from build123d import *

# Parameters (mm, degrees)
CYLINDER001_R     = 1.8
CYLINDER001_DEPTH = 40
ARRAY002_X_COUNT  = 2
ARRAY002_X_PITCH  = 21
CYLINDER002_R     = 1
CYLINDER002_DEPTH = 100
ARRAY003_X_COUNT  = 2
ARRAY003_X_PITCH  = 43
ARRAY003_Y_COUNT  = 2
ARRAY003_Y_PITCH  = 72
CYLINDER003_R     = 1.8
CYLINDER003_DEPTH = 40
ARRAY004_Y_COUNT  = 2
ARRAY004_Y_PITCH  = 71
BOX005_W          = 4
BOX005_H          = 10
BOX005_DEPTH      = 40
CYLINDER004_R     = 2.2
CYLINDER004_DEPTH = 40
ARRAY005_Y_COUNT  = 2
ARRAY005_Y_PITCH  = 34
CYLINDER005_R     = 3
CYLINDER005_DEPTH = 40
CYLINDER_R        = 1.3
CYLINDER_DEPTH    = 40
ARRAY001_X_COUNT  = 2
ARRAY001_X_PITCH  = 19
BOX004_W          = 107
BOX004_H          = 80
BOX004_DEPTH      = 3
FILLET001_R       = 2


with BuildPart() as array002:
    # Cylinder001 → Cylinder001 (new body)
    with BuildSketch(Plane(origin=(75.5, 16.5, -15), x_dir=(1, 0, 0), z_dir=(0, 0, 1))):
        Circle(CYLINDER001_R)
    extrude(amount=CYLINDER001_DEPTH)

    # Array002 X: Array002 ×2


with BuildPart() as array002_1:
    add(array002.part)
    with Locations(*[(i * ARRAY002_X_PITCH, 0, 0) for i in range(1, ARRAY002_X_COUNT)]):
        add(array002.part)


with BuildPart() as array_battery_holder_holes:
    # Cylinder002 → Cylinder002 (new body)
    with BuildSketch(Plane(origin=(13, -4, -15), x_dir=(1, 0, 0), z_dir=(0, 0, 1))):
        Circle(CYLINDER002_R)
    extrude(amount=CYLINDER002_DEPTH)

    # Array003 X: Array battery holder holes ×2


with BuildPart() as array_battery_holder_holes_1:
    add(array_battery_holder_holes.part)
    with Locations(*[(i * ARRAY003_X_PITCH, 0, 0) for i in range(1, ARRAY003_X_COUNT)]):
        add(array_battery_holder_holes.part)

    # Array003 Y: Array battery holder holes ×2


with BuildPart() as array_battery_holder_holes_2:
    add(array_battery_holder_holes_1.part)
    with Locations(*[(0, i * ARRAY003_Y_PITCH, 0) for i in range(1, ARRAY003_Y_COUNT)]):
        add(array_battery_holder_holes_1.part)


with BuildPart() as array_corners:
    # Cylinder003 → Cylinder003 (new body)
    with BuildSketch(Plane(origin=(99, -4.5, -15), x_dir=(1, 0, 0), z_dir=(0, 0, 1))):
        Circle(CYLINDER003_R)
    extrude(amount=CYLINDER003_DEPTH)

    # Array004 Y: Array corners ×2


with BuildPart() as array_corners_1:
    add(array_corners.part)
    with Locations(*[(0, i * ARRAY004_Y_PITCH, 0) for i in range(1, ARRAY004_Y_COUNT)]):
        add(array_corners.part)


with BuildPart() as cube_switch_cut:
    # Box005 → Box005 (new body)
    with BuildSketch(Plane(origin=(78, 1.5, -10), x_dir=(0, -1, 0), z_dir=(0, 0, 1))):
        with Locations((2, 5)):
            Rectangle(BOX005_W, BOX005_H)
    extrude(amount=BOX005_DEPTH)


with BuildPart() as array_usb:
    # Cylinder004 → Cylinder004 (new body)
    with BuildSketch(Plane(origin=(91.5, 24.5, -15), x_dir=(1, 0, 0), z_dir=(0, 0, 1))):
        Circle(CYLINDER004_R)
    extrude(amount=CYLINDER004_DEPTH)

    # Array005 Y: Array usb ×2


with BuildPart() as array_usb_1:
    add(array_usb.part)
    with Locations(*[(0, i * ARRAY005_Y_PITCH, 0) for i in range(1, ARRAY005_Y_COUNT)]):
        add(array_usb.part)


with BuildPart() as cylinder_usb_center:
    # Cylinder005 → Cylinder005 (new body)
    with BuildSketch(Plane(origin=(86, 41.5, -15), x_dir=(1, 0, 0), z_dir=(0, 0, 1))):
        Circle(CYLINDER005_R)
    extrude(amount=CYLINDER005_DEPTH)


with BuildPart() as fusion001:
    # Cylinder → Cylinder (new body)
    with BuildSketch(Plane(origin=(73.5, -0.5, -15), x_dir=(0, -1, 0), z_dir=(0, 0, 1))):
        Circle(CYLINDER_R)
    extrude(amount=CYLINDER_DEPTH)

    # Array001 X: Fusion001 ×2


with BuildPart() as fusion001_1:
    add(fusion001.part)
    with Locations(*[(i * ARRAY001_X_PITCH, 0, 0) for i in range(1, ARRAY001_X_COUNT)]):
        add(fusion001.part)

    # Fusion001: union Array002, Array battery holder holes, Array corners, Cube switch cut, Array usb, Cylinder usb center
    add(array002_1.part)
    add(array_battery_holder_holes_2.part)
    add(array_corners_1.part)
    add(cube_switch_cut.part)
    add(array_usb_1.part)
    add(cylinder_usb_center.part)


with BuildPart() as top_lid_clone:
    # Box004 → Box004 (new body)
    with BuildSketch(Plane(origin=(-3, -8.5, -3), x_dir=(1, 0, 0), z_dir=(0, 0, 1))):
        with Locations((53.5, 40)):
            Rectangle(BOX004_W, BOX004_H)
    extrude(amount=BOX004_DEPTH)

    # Fillet001
    fillet001_edges = [top_lid_clone.edges().sort_by_distance(p)[0] for p in [
        (-3, -8.5, -1.5),
        (-3, 71.5, -1.5),
        (104, -8.5, -1.5),
        (104, 71.5, -1.5),
    ]]
    fillet(fillet001_edges, radius=FILLET001_R)

    # Cut001: cut Fusion001
    add(fusion001_1.part, mode=Mode.SUBTRACT)


solid = top_lid_clone.part
Source: CAD feature listing. Evaluate the final solid. Frame: model axes, mm. A direction names the side the tool comes from. Round coordinates to 2 decimals unless told otherwise and drop trailing zeros. Loops run counter-clockwise (first coordinate to the right, second up) from the corner with the lowest first, then second, coordinate; pieces in that order, holes last. Notation, with made-up numbers: (41, -14) - (75, -14) arc R17 cw to (75, 5) - close; hole circle Ø5 at (44.25, 39.5). An arc over 180 degrees is marked (long way). Write item = value, one per line. Start each with the question number.
Item 1: Reachability of faces 1 (the face through (83, -2.5, -2)), 2 (the face through (50, -8.5, -2)) from +Z, -Z, +X, -X, +Y, -Y: full face, straight path, thin tool, end or side. Return the list, or none.
Item 2: Section query B-B on y = 58.5. Output: boundary loops of the cut face in (x, z), plus the area to 3 significant figures.
Item 3: Material intervals for line 1 (Y direction, x = 99, z = -2.15); line 2 (Y direction, x = 13, z = -2.2); line 3 (Y direction, x = 91.5, z = -1.15), sorted ascending.
Item 4: Mould query, pull axis X, two halves, no side actions, for faces 3 (the face through (-3, 31, -2)), 4 (the face through (91.23, -0.22, -1.52)), 5 (the face through (50, 32, -3)). Classes: released by +X, released by -X, zero draft, split by the parting line, or undercut.
Item 5: Section query C-C on y = 41.5. Output: boundary loops of the cut face in (x, z).
Item 6: Section query A-A on z = -0.5. Count the separate pieces of the cut face and the enclosed holes in it, plus the area to 3 significant figures.
Item 7: First-contact query: pin 1 Ø4 at (x, y) = (99, 66.5) entering from +Z; pin 2 Ø3.5 at (x, y) = (86, 41.5) entering from -Z. Flat tips, straight axial feed; report the tip coordinate or a pass-through.
Results list:
q1.face_1 = +Z, -Z
q1.face_2 = +Z, -Z, +X, -X, -Y
q2.outline = (-3, -3) - (89.3, -3) - (89.3, 0) - (-3, 0) - close; (93.7, -3) - (104, -3) - (104, 0) - (93.7, 0) - close
q2.area = 308 mm²
q3.line_1 = -8.5 to -6.3, -2.7 to 64.7, 68.3 to 71.5
q3.line_2 = -8.5 to -5, -3 to 67, 69 to 71.5
q3.line_3 = -8.5 to -1.33, 0.33 to 22.3, 26.7 to 56.3, 60.7 to 71.5
q4.face_3 = released by -X
q4.face_4 = undercut
q4.face_5 = zero draft
q5.outline = (-3, -3) - (83, -3) - (83, 0) - (-3, 0) - close; (89, -3) - (104, -3) - (104, 0) - (89, 0) - close
q6.separate_pieces = 1
q6.enclosed_holes = 14
q6.area = 8,390 mm²
q7.pin_1 = 0
q7.pin_2 = through
